```python
from build123d import *

# Parameters (mm, degrees)
SKETCH1_R               = 1.3
BOSS_EXTRUDE1_DEPTH     = 32.8
CHAMFER1_SIZE           = 1.9
CHAMFER2_SIZE           = 1.9
SKETCH2_R               = 6
BOSS_EXTRUDE2_DEPTH     = 22
SKETCH3_R               = 1.3
CUT_EXTRUDE1_DEPTH      = 1
CUT_EXTRUDE1_DEPTH_BACK = 23


with BuildPart() as part:
    # Sketch1 → Boss-Extrude1 (new body)
    with BuildSketch(Plane(origin=(0, 0, 0), x_dir=(1, 0, 0), z_dir=(0, 1, 0))):
        Polygon((-1.5, 0), (-7.5, 0), (-7.5, -22), (7.5, -22), (7.5, 0), (1.5, 0), (1.5, -8.5), (-1.5, -8.5), align=None)
        with Locations((0, -17)):
            Circle(SKETCH1_R, mode=Mode.SUBTRACT)
        with Locations((0, -12)):
            Circle(SKETCH1_R, mode=Mode.SUBTRACT)
    extrude(amount=BOSS_EXTRUDE1_DEPTH)

    # Chamfer1
    chamfer1_edges = [part.edges().sort_by_distance(p)[0] for p in [
        (7.5, 0, 11),
        (7.5, 32.8, 11),
    ]]
    chamfer(chamfer1_edges, length=CHAMFER1_SIZE)

    # Chamfer2
    chamfer2_edges = [part.edges().sort_by_distance(p)[0] for p in [
        (-7.5, 0, 11),
        (-7.5, 32.8, 11),
    ]]
    chamfer(chamfer2_edges, length=CHAMFER2_SIZE)

    # Sketch2 → Boss-Extrude2 (add)
    with BuildSketch(Plane(origin=(0, 0, 0), x_dir=(-1, 0, 0), z_dir=(0, 0, -1))):
        with Locations((7.5, 16.4)):
            Circle(SKETCH2_R)
    extrude(amount=-BOSS_EXTRUDE2_DEPTH)

    # Sketch3 → Cut-Extrude1 (cut, two sides)
    with BuildSketch(Plane(origin=(0, 0, 0), x_dir=(-1, 0, 0), z_dir=(0, 0, -1))) as cut_extrude1_sk:
        with Locations((7.5, 16.4)):
            Circle(SKETCH3_R)
    extrude(amount=CUT_EXTRUDE1_DEPTH, mode=Mode.SUBTRACT)
    extrude(cut_extrude1_sk.sketch, amount=-CUT_EXTRUDE1_DEPTH_BACK, mode=Mode.SUBTRACT)


solid = part.part
```
Can you work these out from the model? Positions are in its coordinate system, mm. A direction names the side the tool comes from. Coordinates: 2 decimals unless noted, no trailing zeros. Loops run counter-clockwise (first coordinate to the right, second up) from the corner with the lowest first, then second, coordinate; pieces in that order, holes last.
1) For pin 1 (2.5 mm diameter, centred on x = -7.5, y = 16.4, fed in from +Z); pin 2 (5 mm diameter, centred on x = -10.5, z = 12, fed in from -Y); pin 3 (4 mm diameter, centred on y = 26, z = 16, fed in from -X); pin 4 (4 mm diameter, centred on y = 12, z = 3.5, fed in from -X), each with a flat end and sliding along its axis, tell me the tip position at first contact or that it passes through.
2) Imagine slicing it at B-B on z = 17. List the corners of the cut face in (x, y) for me.
3) Imagine slicing it at A-A on y = 16.4. List the corners of the cut face in (x, z) for me.
4) Which directions (+Z, -Z, +X, -X, +Y, -Y) give clear straight access to the entire face, cutting with the end or side of a thin tool? Please do faces 1 (the flat face through (-1.5, 16, 4)), 2 (the flat face through (-7.5, 6, 11)), 3 (the cylindrical face through (-13.5, 16.3, 10.8)), 4 (the flat face through (1.2, 0, 10.8)), 5 (the flat face through (-7.5, 27, 11)).
5) I need wall thicknesses on probe 1 along Z at (x, y) = (0, 23); probe 2 along X at (y, z) = (8.5, 6.25); probe 3 along Z at (x, y) = (0.5, 28.5). Which ranges of each line are inside material? Lowest first, please.
6) Imagine slicing it at D-D on z = 9.5. List the corners of the cut face in (x, y) for me, plus the area to 3 significant figures.
7) Imagine slicing it at C-C on x = 0. List the corners of the cut face in (y, z) for me.
8) Thinking about a two-plate mould opening in Z: for faces 6 (the flat face through (5, 16, 0)), 7 (the cylindrical face through (-0.17, 16.17, 15.71)), 8 (the flat face through (6.5, 0.9, 11.2)), which applies, pulls with the +Z half, pulls with the -Z half, needs draft (parallel to the pull), parting line crosses it, or undercut?
Completed:
1. pin 1: passes through
1. pin 2: stops at y = 10.42
1. pin 3: stops at x = -7.5
1. pin 4: stops at x = -13
2. outline: (-7.5, 1.9) - (-5.6, 0) - (-1.3, 0) - (-1.3, 32.8) - (-5.6, 32.8) - (-7.5, 30.9) - (-7.5, 22.4) arc R6 ccw to (-7.5, 10.4) - close; (1.3, 0) - (5.6, 0) - (7.5, 1.9) - (7.5, 30.9) - (5.6, 32.8) - (1.3, 32.8) - close; hole circle Ø2.6 at (-7.5, 16.4)
3. outline: (-13.5, 0) - (-8.8, 0) - (-8.8, 22) - (-13.5, 22) - close; (-6.2, 0) - (-1.5, 0) - (-1.5, 8.5) - (1.5, 8.5) - (1.5, 0) - (7.5, 0) - (7.5, 22) - (-6.2, 22) - close; hole circle Ø2.6 at (0, 12); hole circle Ø2.6 at (0, 17)
4. face 1: -Z, +Y, -Y
4. face 2: +Z, -Z, -X, -Y
4. face 3: +Z, -Z, -X
4. face 4: +Z, -Z, +X, -X, -Y
4. face 5: +Z, -Z, -X, +Y
5. probe 1: z = 8.5 to 10.7, 13.3 to 15.7, 18.3 to 22
5. probe 2: x = -7.5 to -1.5, 1.5 to 7.5
5. probe 3: z = 8.5 to 10.8, 13.2 to 15.8, 18.2 to 22
6. outline: (-7.5, 1.9) - (-5.6, 0) - (5.6, 0) - (7.5, 1.9) - (7.5, 30.9) - (5.6, 32.8) - (-5.6, 32.8) - (-7.5, 30.9) - (-7.5, 22.4) arc R6 ccw to (-7.5, 10.4) - close; hole circle Ø2.6 at (-7.5, 16.4)
6. area: 536 mm2
7. outline: (0, 8.5) - (32.8, 8.5) - (32.8, 10.7) - (0, 10.7) - close; (0, 13.3) - (32.8, 13.3) - (32.8, 15.7) - (0, 15.7) - close; (0, 18.3) - (32.8, 18.3) - (32.8, 22) - (0, 22) - close
8. face 6: pulls with the -Z half
8. face 7: undercut
8. face 8: needs draft
